The model under review builds one solid part; all positions refer to its coordinate system, in mm. Face numbers are marked on the shaded views. Coordinates: 2 decimals unless noted, no trailing zeros. Write each loop counter-clockwise with the first axis right and the second up, starting at its lowest first coordinate (ties: lowest second). Pieces come first, ordered by that corner, then holes. Notation, with made-up numbers: (34, 56) - (83, 56) arc R21 ccw to (83, 93) - close; hole circle Ø4 at (-36, 78.5). An arc over 180 degrees is marked (long way). Put each result on its own line as item: value. Start each with the question number.
Item 1: Consider section A-A on y = 0. Give the boundary of the cut face in (x, z) (3 decimals).
Item 2: Consider section D-D on y = 47. Give the boundary of the cut face in (x, z) (3 decimals), then the cut area to 3 significant figures.
Item 3: Mouldability with a two-part tool opening along Y and no side actions: class the marked faces 1, 2 and 3 as pulls with the +Y half, pulls with the -Y half, needs draft (parallel to the pull), parting line crosses it, or undercut.
Item 4: Consider section C-C on x = 0. Give the boundary of the cut face in (y, z) (3 decimals).
Item 5: For pin 1 (10 mm diameter, centred on y = -66, z = 107, fed in from +X); pin 2 (3 mm diameter, centred on x = 58.5, z = 250, fed in from -Y); pin 3 (10 mm diameter, centred on y = 0, z = 279.4, fed in from -X); pin 4 (12 mm diameter, centred on x = 64, z = 156, fed in from -Y), all flat-tipped, find the tip position at first contact; note any pin that passes through.
Item 6: Consider section B-B on z = 127. Give the boundary of the cut face in (x, y) (3 decimals).
Item 7: To check wall thickness, follow L1, parallel to Z at x = 99.65, y = 0; L2, parallel to Y at x = 0, z = 128.5 (3 decimals); L3, parallel to Z at x = -5.5, y = 28 (3 decimals). State the ranges of each line that lie inside material, in increasing order. Write a range as [from, to].
```python
from build123d import *

# Parameters (mm, degrees)
F0_R     = 101.6
F1_DEPTH = 304.8
F2_T     = -3.175
F3_R     = 6.35
F4_DEPTH = 279.4


with BuildPart() as f1:
    # F0 (on Top) → F1 (new body)
    with BuildSketch(Plane.XY):
        Circle(F0_R)
    extrude(amount=F1_DEPTH)

    # F2
    f2_openings = [f1.faces().sort_by_distance(p)[0] for p in [
        (0, 0, 304.8),
    ]]
    offset(amount=F2_T, openings=f2_openings)

    # F3 (on Right) → F4 (cut, symmetric)
    with BuildSketch(Plane.YZ):
        with Locations((0, 279.4)):
            Circle(F3_R)
        with Locations((0, 127)):
            Circle(F3_R)
    extrude(amount=F4_DEPTH, both=True, mode=Mode.SUBTRACT)


solid = f1.part
```
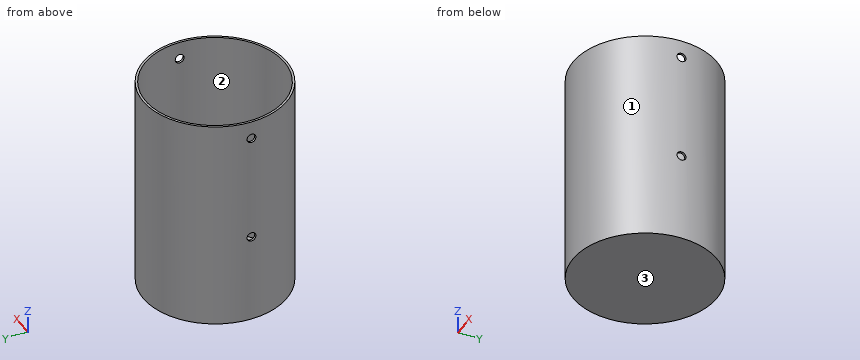
Report:
1. outline: (-101.6, 0) - (101.6, 0) - (101.6, 120.65) - (98.425, 120.65) - (98.425, 3.175) - (-98.425, 3.175) - (-98.425, 120.65) - (-101.6, 120.65) - close; (-101.6, 133.35) - (-98.425, 133.35) - (-98.425, 273.05) - (-101.6, 273.05) - close; (-101.6, 285.75) - (-98.425, 285.75) - (-98.425, 304.8) - (-101.6, 304.8) - close; (98.425, 133.35) - (101.6, 133.35) - (101.6, 273.05) - (98.425, 273.05) - close; (98.425, 285.75) - (101.6, 285.75) - (101.6, 304.8) - (98.425, 304.8) - close
2. outline: (-90.075, 0) - (90.075, 0) - (90.075, 304.8) - (86.478, 304.8) - (86.478, 3.175) - (-86.478, 3.175) - (-86.478, 304.8) - (-90.075, 304.8) - close
2. area: 2,740 mm²
3. face 1: parting line crosses it
3. face 2: undercut
3. face 3: needs draft
4. outline: (-101.6, 0) - (101.6, 0) - (101.6, 304.8) - (98.425, 304.8) - (98.425, 3.175) - (-98.425, 3.175) - (-98.425, 304.8) - (-101.6, 304.8) - close
5. pin 1: x = 81.25
5. pin 2: y = -84.1
5. pin 3: through
5. pin 4: y = -83.42
6. outline: (-101.401, -6.35) arc R101.6 ccw to (101.401, -6.35) - (98.22, -6.35) arc R98.425 cw to (-98.22, -6.35) - close; (-101.401, 6.35) - (-98.22, 6.35) arc R98.425 cw to (98.22, 6.35) - (101.401, 6.35) arc R101.6 ccw to start
7. L1: [0, 120.65], [133.35, 273.05], [285.75, 304.8]
7. L2: [-101.6, -98.425], [98.425, 101.6]
7. L3: [0, 3.175]
